Can you work these out from the model? Positions are in its coordinate system, mm. Face numbers are marked on the shaded views. A direction names the side the tool comes from. Round coordinates to 2 decimals unless told otherwise and drop trailing zeros. Write each loop counter-clockwise with the first axis right and the second up, starting at its lowest first coordinate (ties: lowest second). Pieces come first, ordered by that corner, then holes.
Q1. I'm going to push flat-ended pins straight in: pin 1 Ø1.5 at (x, y) = (249, 50.5) entering from -Z; pin 2 Ø0.9 at (x, y) = (248.5, 47) entering from +Z; pin 3 Ø3.5 at (y, z) = (572, -148.5) entering from -X. Where does each tip first touch, or does it pass through?
Q2. If we section it at A-A (z = -107.5): Please give me the cut outline in (x, y), plus the area to 3 significant figures.
Q3. If we section it at C-C (z = -73): Please give me the cut outline in (x, y).
Q4. If we section it at B-B (x = 68): Please give me the cut outline in (y, z).
Q5. For the marked faces 1 and 2, which set-ups out of +Z, -Z, +X, -X, +Y, -Y let a thin tool reach every point of the face, with its end or its side?
Q6. Please list where these lines run through material, in increasing order: line 1 along Y through (x, z) = (233, -148.2); line 2 along X through (y, z) = (72, -123.5); line 3 along Z through (x, y) = (122, 58).
Q7. If we section it at D-D (y = 369): Please give me the cut outline in (x, z), plus the area to 3 significant figures.
Q8. We'd pull the mould along Z, two halves only. Please class the marked faces 3, 4 and 5: +Z half, -Z half, draft (parallel to the pull), parting line (faces both ways), or undercut.
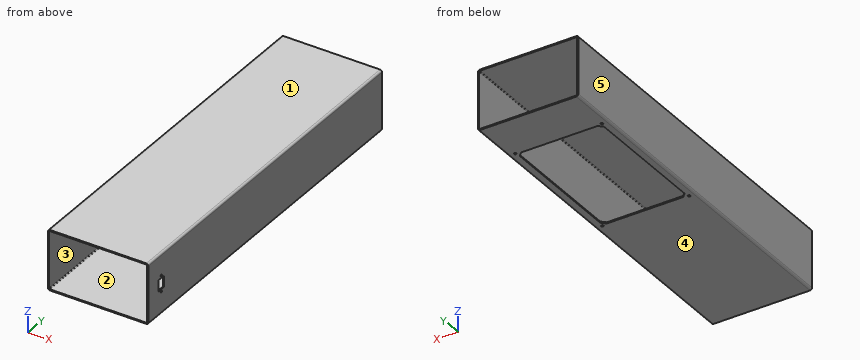
from build123d import *

# Parameters (mm, degrees)
ESQUISSE1_W             = 250
ESQUISSE1_H             = 150
BASE_EXTRUSION_DEPTH    = 900
CONG_2_R                = 5
COQUE1_T                = -3
ENL_V_MAT_EXTRU_2_DEPTH = 10
ESQUISSE4_R             = 3
ENL_V_MAT_EXTRU_3_DEPTH = 10
ESQUISSE6_R             = 2.5
ESQUISSE6_W             = 28
ESQUISSE6_H             = 21
ENL_V_MAT_EXTRU_4_DEPTH = 8


with BuildPart() as part:
    # Esquisse1 → Base-Extrusion (new body)
    with BuildSketch(Plane(origin=(0, 0, 0), x_dir=(1, 0, 0), z_dir=(0, 1, 0))):
        with Locations((125, 75)):
            Rectangle(ESQUISSE1_W, ESQUISSE1_H)
    extrude(amount=BASE_EXTRUSION_DEPTH)

    # Congé2
    cong_2_edges = [part.edges().sort_by_distance(p)[0] for p in [
        (0, 450, 0),
        (250, 450, 0),
        (250, 450, -150),
        (0, 450, -150),
    ]]
    fillet(cong_2_edges, radius=CONG_2_R)

    # Coque1
    coque1_openings = [part.faces().sort_by_distance(p)[0] for p in [
        (125, 0, -75),
        (125, 900, -75),
    ]]
    offset(amount=COQUE1_T, openings=coque1_openings, kind=Kind.INTERSECTION)

    # Esquisse3 → Enlèv. mat.-Extru.2 (cut)
    with BuildSketch(Plane(origin=(0, 0, -150), x_dir=(-1, 0, 0), z_dir=(0, 0, -1))):
        Polygon((-230, 770), (-220, 780), (-30, 780), (-20, 770), (-20, 460), (-30, 450), (-220, 450), (-230, 460), align=None)
    extrude(amount=-ENL_V_MAT_EXTRU_2_DEPTH, mode=Mode.SUBTRACT)

    # Esquisse4 → Enlèv. mat.-Extru.3 (cut)
    with BuildSketch(Plane(origin=(0, 0, -150), x_dir=(-1, 0, 0), z_dir=(0, 0, -1))):
        with Locations(Location((-17, 783, 0), (0, 0, 90))):
            Circle(ESQUISSE4_R)
        with Locations(Location((-17, 447, 0), (0, 0, 90))):
            Circle(ESQUISSE4_R)
        with Locations(Location((-233, 783, 0), (0, 0, 90))):
            Circle(ESQUISSE4_R)
        with Locations(Location((-233, 447, 0), (0, 0, 90))):
            Circle(ESQUISSE4_R)
    extrude(amount=-ENL_V_MAT_EXTRU_3_DEPTH, mode=Mode.SUBTRACT)

    # Esquisse6 → Enlèv. mat.-Extru.4 (cut)
    with BuildSketch(Plane(origin=(250, 0, 0), x_dir=(0, 0, -1), z_dir=(1, 0, 0))):
        with Locations(Location((95, 50, 0), (0, 0, 90))):
            Circle(ESQUISSE6_R)
        with Locations(Location((55, 50, 0), (0, 0, 90))):
            Circle(ESQUISSE6_R)
        with Locations((75, 50)):
            Rectangle(ESQUISSE6_W, ESQUISSE6_H)
    extrude(amount=-ENL_V_MAT_EXTRU_4_DEPTH, mode=Mode.SUBTRACT)


solid = part.part
A:
1. pin 1: stops at z = -148.8
1. pin 2: stops at z = -1.04
1. pin 3: stops at x = 0.32
2. outline: (0, 0) - (3, 0) - (3, 900) - (0, 900) - close; (247, 0) - (250, 0) - (250, 900) - (247, 900) - close
2. area: 5,400 mm2
3. outline: (0, 0) - (3, 0) - (3, 900) - (0, 900) - close; (247, 0) - (250, 0) - (250, 39.5) - (247, 39.5) - close; (247, 60.5) - (250, 60.5) - (250, 900) - (247, 900) - close
4. outline: (0, -150) - (450, -150) - (450, -147) - (0, -147) - close; (0, -3) - (900, -3) - (900, 0) - (0, 0) - close; (780, -150) - (900, -150) - (900, -147) - (780, -147) - close
5. face 1: +Z, +X, -X, +Y, -Y
5. face 2: +Y, -Y
6. line 1: y = 0 to 444, 450 to 780, 786 to 900
6. line 2: x = 0 to 3, 247 to 250
6. line 3: z = -150 to -147, -3 to 0
7. outline: (0, -145) arc R5 ccw to (5, -150) - (245, -150) arc R5 ccw to (250, -145) - (250, -5) arc R5 ccw to (245, 0) - (5, 0) arc R5 ccw to (0, -5) - close; hole (3, -145) arc R2 ccw to (5, -147) - (245, -147) arc R2 ccw to (247, -145) - (247, -5) arc R2 ccw to (245, -3) - (5, -3) arc R2 ccw to (3, -5) - close
7. area: 2,350 mm2
8. face 3: undercut
8. face 4: -Z half
8. face 5: draft
